from build123d import *

# Parameters (mm, degrees)
F1_DEPTH = 10


with BuildPart() as f1:
    # F0 (on Front) → F1 (new body)
    with BuildSketch(Plane.XZ):
        with BuildLine():
            ThreePointArc((-90, 43.5889894354), (-70.7106781187, 70.7106781187), (-43.5889894354, 90))
            Line((-43.5889894354, 90), (-78, 90))
            ThreePointArc((-78, 90), (-86.4852813742, 86.4852813742), (-90, 78))
            Line((-90, 78), (-90, 43.5889894354))
        make_face()
        with BuildLine():
            Line((-43.5889894354, 90), (43.5889894354, 90))
            ThreePointArc((43.5889894354, 90), (0, 100), (-43.5889894354, 90))
        make_face()
        with BuildLine():
            ThreePointArc((43.5889894354, 90), (70.7106781187, 70.7106781187), (90, 43.5889894354))
            Line((90, 43.5889894354), (90, 78))
            ThreePointArc((90, 78), (86.4852813742, 86.4852813742), (78, 90))
            Line((78, 90), (43.5889894354, 90))
        make_face()
        with BuildLine():
            Line((90, -78), (90, -43.5889894354))
            ThreePointArc((90, -43.5889894354), (70.7106781187, -70.7106781187), (43.5889894354, -90))
            Line((43.5889894354, -90), (78, -90))
            ThreePointArc((78, -90), (86.4852813742, -86.4852813742), (90, -78))
        make_face()
        with BuildLine():
            Line((-78, -90), (-43.5889894354, -90))
            ThreePointArc((-43.5889894354, -90), (-70.7106781187, -70.7106781187), (-90, -43.5889894354))
            Line((-90, -43.5889894354), (-90, -78))
            ThreePointArc((-90, -78), (-86.4852813742, -86.4852813742), (-78, -90))
        make_face()
        with BuildLine():
            Line((90, -43.5889894354), (90, 43.5889894354))
            ThreePointArc((90, 43.5889894354), (70.7106781187, 70.7106781187), (43.5889894354, 90))
            Line((43.5889894354, 90), (-43.5889894354, 90))
            ThreePointArc((-43.5889894354, 90), (-70.7106781187, 70.7106781187), (-90, 43.5889894354))
            Line((-90, 43.5889894354), (-90, -43.5889894354))
            ThreePointArc((-90, -43.5889894354), (-70.7106781187, -70.7106781187), (-43.5889894354, -90))
            Line((-43.5889894354, -90), (43.5889894354, -90))
            ThreePointArc((43.5889894354, -90), (70.7106781187, -70.7106781187), (90, -43.5889894354))
        make_face()
        with BuildLine():
            Line((-90, -43.5889894354), (-90, 43.5889894354))
            ThreePointArc((-90, 43.5889894354), (-100, 0), (-90, -43.5889894354))
        make_face()
        with BuildLine():
            ThreePointArc((-43.5889894354, -90), (0, -100), (43.5889894354, -90))
            Line((43.5889894354, -90), (-43.5889894354, -90))
        make_face()
        with BuildLine():
            ThreePointArc((90, -43.5889894354), (97.4679434481, -22.360679775), (100, 0))
            ThreePointArc((100, 0), (97.4679434481, 22.360679775), (90, 43.5889894354))
            Line((90, 43.5889894354), (90, -43.5889894354))
        make_face()
    extrude(amount=F1_DEPTH)


solid = f1.part
Work out the finished part from the listing and answer in its coordinate system (mm). A direction names the side the tool comes from. Coordinates: 2 decimals unless noted, no trailing zeros. Loops run counter-clockwise (first coordinate to the right, second up) from the corner with the lowest first, then second, coordinate; pieces in that order, holes last. Notation, with made-up numbers: M 10.25,48 L 63.25,48 A12 ccw 63.25,52 Z; hole C 21,13 d9. An arc over 180 degrees is marked long. Answer in a Markdown table with one row per item. Add a question column.
1. Find section C-C, the plane z = -46.5. Write down the section's boundary in (x, y).
2. Consider L1, parallel to Z at x = -75.5, y = -2.75; L2, parallel to X at y = -9, z = -1 (3 decimals). Determine where each line is inside the solid, lowest interval first.
3. Flat-ended cylindrical pins translate along their axes: P1, Ø1.5, axis at y = -7, z = -33.5, coming from the +X side; P2, Ø3, axis at x = -59.5, y = -5.5, coming from the +Z side; P3, Ø4, axis at x = 77, y = -3.5, coming from the -Z side. Find the tip coordinate at first contact, or state that the pin passes through.
4. Find section A-A, the plane y = -1.75. Write down the section's boundary in (x, z).
5. A tool of negligible diameter and unlimited length cuts with its end or side. For faces 1 (the flat face through (-61, -5, 90)), 2 (the flat face through (-90, -5, -61)), 3 (the flat face through (61, -5, 90)), from which of +Z, -Z, +X, -X, +Y, -Y can it reach the whole face along a straight path? Write none if from no direction.
6. Find section B-B, the plane x = -69. Write down the section's boundary in (y, z).
Reported:
| question | item | result |
|---|---|---|
| 1 | outline | M -90,-10 L 90,-10 L 90,0 L -90,0 Z |
| 2 | L1 | z = -90 to 90 |
| 2 | L2 | x = -99.995 to 99.995 |
| 3 | P1 | stops at x = 94.49 |
| 3 | P2 | stops at z = 90 |
| 3 | P3 | stops at z = -90 |
| 4 | outline | M -90,-78 A12 ccw -78,-90 L -43.59,-90 A100 ccw 43.59,-90 L 78,-90 A12 ccw 90,-78 L 90,-43.59 A100 ccw 90,43.59 L 90,78 A12 ccw 78,90 L 43.59,90 A100 ccw -43.59,90 L -78,90 A12 ccw -90,78 L -90,43.59 A100 ccw -90,-43.59 Z |
| 5 | face 1 | +Z, -X, +Y, -Y |
| 5 | face 2 | -Z, -X, +Y, -Y |
| 5 | face 3 | +Z, +X, +Y, -Y |
| 6 | outline | M -10,-90 L 0,-90 L 0,90 L -10,90 Z |
